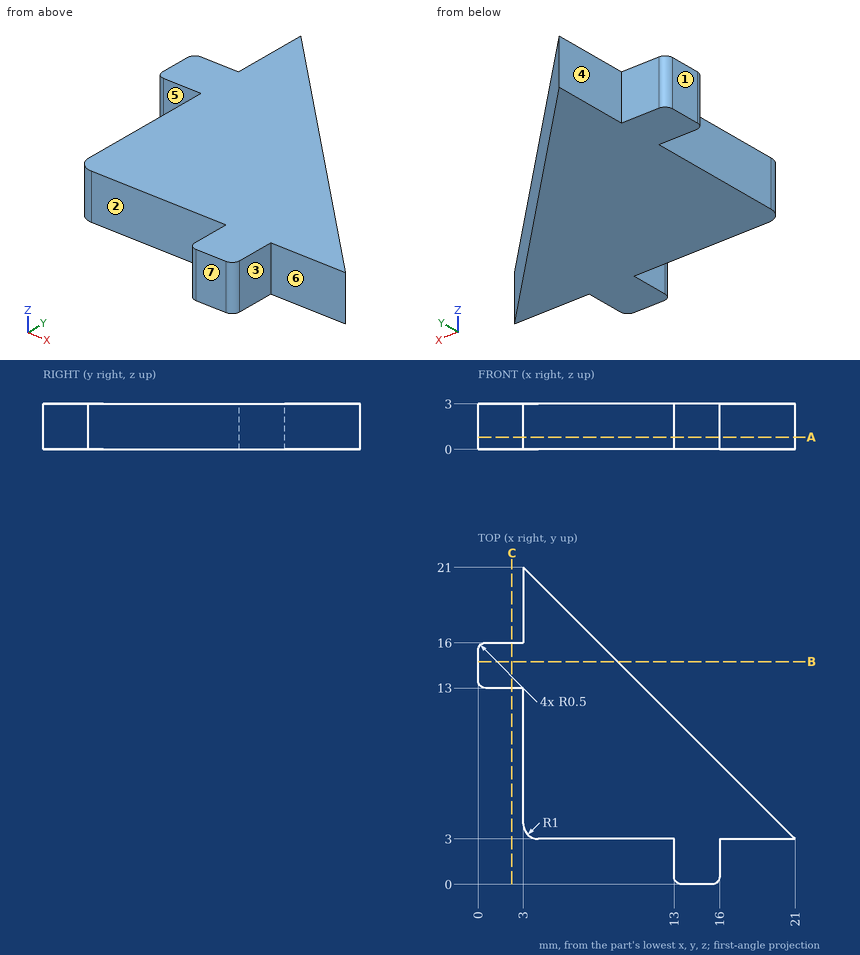
Could you check a few things on this drawing? It's one solid part, dimensions in mm from its lowest x, y, z. A direction names the side the tool comes from. Give positions to 0.01 mm unless a question says otherwise; leave off trailing zeros. Order: outer loops, then holes, each group sorted by start corner. A loop starts at its lowest first (then second) coordinate and runs counter-clockwise, first axis right, second up. Notation, with made-up numbers: (3, 56.5) - (30, 56.5) arc R18 ccw to (30, 61.5) - close; hole circle Ø7 at (16.25, 25.25). An arc over 180 degrees is marked (long way). One line per item, written item: value. Start each with the question number.
1. Imagine slicing it at B-B on y = 14.75. List the corners of the cut face in (x, z) for me.
2. For P1, Ø8, axis at x = 3, y = 5, coming from the -Z side; P2, Ø1.2, axis at y = 2, z = 1.5, coming from the -X side; P3, Ø1.5, axis at y = 8, z = 2, coming from the -X side; P4, Ø1.2, axis at y = 2, z = 1, coming from the +X side, each with a flat end and sliding along its axis, tell me the tip position at first contact or that it passes through.
3. Imagine slicing it at C-C on x = 2.25. List the corners of the cut face in (y, z) for me.
4. If I drill on probe 1 along X at (y, z) = (1, 2.3); probe 2 along X at (y, z) = (13.5, 2.3), over which ranges is the centre line in solid material (lowest first)?
5. Imagine slicing it at A-A on z = 0.8. List the corners of the cut face in (x, y) for me, plus the area to 3 significant figures.
6. For the marked faces 4, 5, 6 and 7, which set-ups out of +Z, -Z, +X, -X, +Y, -Y let a thin tool reach every point of the face, with its end or its side?
7. Thinking about a two-plate mould opening in X: for the marked faces 1, 2 and 3, which applies, +X half, -X half, draft (parallel to the pull), parting line (faces both ways), or undercut?
Values:
1. outline: (0, 0) - (9.25, 0) - (9.25, 3) - (0, 3) - close
2. P1: z = 0
2. P2: x = 13
2. P3: x = 3
2. P4: x = 16
3. outline: (13, 0) - (16, 0) - (16, 3) - (13, 3) - close
4. probe 1: 13 to 16
4. probe 2: 0 to 10.5
5. outline: (0, 13.5) arc R0.5 ccw to (0.5, 13) - (3, 13) - (3, 4) arc R1 ccw to (4, 3) - (13, 3) - (13, 0.5) arc R0.5 ccw to (13.5, 0) - (15.5, 0) arc R0.5 ccw to (16, 0.5) - (16, 3) - (21, 3) - (3, 21) - (3, 16) - (0.5, 16) arc R0.5 ccw to (0, 15.5) - close
5. area: 180 mm²
6. face 4: +Z, -Z, -X, +Y
6. face 5: +Z, -Z, -X, -Y
6. face 6: +Z, -Z, +X, -Y
6. face 7: +Z, -Z, +X, -X, -Y
7. face 1: -X half
7. face 2: draft
7. face 3: +X half
